from build123d import *

# Parameters (mm, degrees)
SKETCH2_R           = 1.4
SKETCH2_R_2         = 1.65
BOSS_EXTRUDE1_DEPTH = 4.7
SKETCH3_R           = 4.5
SKETCH3_R_2         = 1.65
BOSS_EXTRUDE2_DEPTH = 2
FILLET1_R           = 5
CHAMFER1_SIZE       = 3
CUT_EXTRUDE1_DEPTH  = 3
BOSS_EXTRUDE3_START = -4.7
SKETCH5_R           = 1.4
BOSS_EXTRUDE3_DEPTH = 4.7
BOSS_EXTRUDE4_START = 2.7
SKETCH6_W           = 17.015251106
SKETCH6_H           = 6.441411174
SKETCH6_R           = 1.4
BOSS_EXTRUDE4_DEPTH = 2.7


with BuildPart() as part:
    # Sketch2 → Boss-Extrude1 (new body)
    with BuildSketch(Plane.XY):
        with BuildLine():
            Line((5.681498191, -33.388801204), (5.681498191, -42.638801204))
            Line((5.681498191, -42.638801204), (-15.818501809, -42.638801204))
            Line((-15.818501809, -42.638801204), (-15.818501809, -40.088801204))
            ThreePointArc((-15.818501809, -40.088801204), (-17.282967903, -36.553267298), (-20.818501809, -35.088801204))
            Line((-20.818501809, -35.088801204), (-32.818501809, -35.088801204))
            Line((-32.818501809, -35.088801204), (-32.818501809, -4.488801204))
            Line((-32.818501809, -4.488801204), (-12.818501809, -4.488801204))
            Line((-12.818501809, -4.488801204), (-3.637114605, -4.488801204))
            Line((-3.637114605, -4.488801204), (-3.637114605, -4.888801204))
            Line((-3.637114605, -4.888801204), (-3.637114605, -9.488801204))
            Line((-3.637114605, -9.488801204), (-3.637114605, -33.388801204))
            Line((-3.637114605, -33.388801204), (5.681498191, -33.388801204))
        make_face()
        with Locations((-8.237114605, -14.488801204)):
            Circle(SKETCH2_R, mode=Mode.SUBTRACT)
        with Locations((0.681498191, -37.638801204)):
            Circle(SKETCH2_R_2, mode=Mode.SUBTRACT)
        with BuildLine():
            ThreePointArc((-27.418501809, -27.538801204), (-26.510532831, -29.730832226), (-24.318501809, -30.638801204))
            ThreePointArc((-24.318501809, -30.638801204), (-22.126470787, -25.346770182), (-27.418501809, -27.538801204))
        make_face(mode=Mode.SUBTRACT)
        with BuildLine():
            ThreePointArc((-13.418501809, -27.538801204), (-12.510532831, -29.730832226), (-10.318501809, -30.638801204))
            ThreePointArc((-10.318501809, -30.638801204), (-8.126470787, -25.346770182), (-13.418501809, -27.538801204))
        make_face(mode=Mode.SUBTRACT)
    extrude(amount=BOSS_EXTRUDE1_DEPTH)

    # Sketch3 → Boss-Extrude2 (add)
    # profile 1 of 2: a face of its own
    with BuildSketch(Plane.XY.offset(4.7)):
        with Locations((-24.318501809, -27.538801204)):
            Circle(SKETCH3_R)
        with Locations((-24.318501809, -27.538801204)):
            Circle(SKETCH3_R_2, mode=Mode.SUBTRACT)
    # profile 2 of 2: a face of its own
    with BuildSketch(Plane.XY.offset(4.7)):
        with Locations((-10.318501809, -27.538801204)):
            Circle(SKETCH3_R)
        with Locations((-10.318501809, -27.538801204)):
            Circle(SKETCH3_R_2, mode=Mode.SUBTRACT)
    extrude(amount=BOSS_EXTRUDE2_DEPTH)

    # Fillet1
    fillet1_edges = [part.edges().sort_by_distance(p)[0] for p in [
        (-15.818501809, -42.638801204, 2.35),
        (-32.818501809, -35.088801204, 2.35),
        (-32.818501809, -4.488801204, 2.35),
    ]]
    fillet(fillet1_edges, radius=FILLET1_R)

    # Chamfer1
    chamfer1_edges = [part.edges().sort_by_distance(p)[0] for p in [
        (5.681498191, -33.388801204, 2.35),
        (5.681498191, -42.638801204, 2.35),
    ]]
    chamfer(chamfer1_edges, length=CHAMFER1_SIZE)

    # Sketch4 → Cut-Extrude1 (cut)
    with BuildSketch(Plane.XY.offset(4.7)):
        Polygon((-3.637114605, -42.638801204), (2.681498191, -42.638801204), (5.681498191, -39.638801204), (5.681498191, -36.388801204), (2.681498191, -33.388801204), (-3.637114605, -33.388801204), align=None)
        Polygon((-3.637114605, -9.488801204), (-10.237114605, -9.488801204), (-13.237114605, -12.488801204), (-13.237114605, -16.488801204), (-10.237114605, -19.488801204), (-3.637114605, -19.488801204), align=None)
    extrude(amount=-CUT_EXTRUDE1_DEPTH, mode=Mode.SUBTRACT)

    # Sketch5 → Boss-Extrude3 (add)
    with BuildSketch(Plane(origin=(0, 0, 0), x_dir=(-1, 0, 0), z_dir=(0, 0, -1)).offset(BOSS_EXTRUDE3_START)):
        with BuildLine():
            Line((12.803250703, -4.488801204), (12.803250703, 3.75260997))
            Line((12.803250703, 3.75260997), (30.118597337, 3.75260997))
            Line((30.118597337, 3.75260997), (32.818501809, -2.119551062))
            Line((32.818501809, -2.119551062), (32.818501809, -9.488801204))
            ThreePointArc((32.818501809, -9.488801204), (31.354035715, -5.953267298), (27.818501809, -4.488801204))
            Line((27.818501809, -4.488801204), (12.803250703, -4.488801204))
        make_face()
        with Locations((26.568501809, 1.011198796)):
            Circle(SKETCH5_R, mode=Mode.SUBTRACT)
        with Locations((16.068501809, 1.011198796)):
            Circle(SKETCH5_R, mode=Mode.SUBTRACT)
    extrude(amount=BOSS_EXTRUDE3_DEPTH)

    # Sketch6 → Boss-Extrude4 (add)
    with BuildSketch(Plane.XY.offset(4.7).offset(BOSS_EXTRUDE4_START)):
        with Locations((-21.310876256, 0.531904383)):
            Rectangle(SKETCH6_W, SKETCH6_H)
        with Locations(Location((-26.568501809, 1.011198796, 0), (0, 0, 180))):
            Circle(SKETCH6_R, mode=Mode.SUBTRACT)
        with Locations(Location((-16.068501809, 1.011198796, 0), (0, 0, 180))):
            Circle(SKETCH6_R, mode=Mode.SUBTRACT)
    extrude(amount=-BOSS_EXTRUDE4_DEPTH)


solid = part.part
Check sheet for the modelled part. Datum: model origin and axes. Units: mm. A direction names the side the tool comes from. Give positions to 0.01 mm unless a question says otherwise; leave off trailing zeros. Loops run counter-clockwise (first coordinate to the right, second up) from the corner with the lowest first, then second, coordinate; pieces in that order, holes last. Notation, with made-up numbers: M 38,22.25 L 81,22.25 A27 cw 81,61.25 Z; hole C 17,34.5 d6. An arc over 180 degrees is marked long. Return JSON: item names as keys, results as strings. Group by question number.
1. Cross-section at C-C on y = -6. Record the boundary of the cut face in (x, z).
2. Thickness scan on L1, parallel to X at y = 1.5, z = 4.25; L2, parallel to X at y = -29, z = 4.75; L3, parallel to Y at x = -13, z = 3. Record the ranges inside material, lowest first.
3. Go/stop test with flat-tipped pins: pin 1 (10 mm diameter, centred on x = -5.5, y = -4, fed in from -Z); pin 2 (2.5 mm diameter, centred on x = -24, y = -29.5, fed in from +Z); pin 3 (3 mm diameter, centred on y = -21, z = 5, fed in from +X); pin 4 (4 mm diameter, centred on x = -24, z = 1.5, fed in from -Y). Record where each tip stops, or that it passes through.
4. Tool access check on faces 4 (the flat face through (-11.72, -10.97, 3.22)), 5 (the flat face through (-12.803, 0, 4)), 6 (the flat face through (-24, -35.089, 2)), 7 (the flat face through (2, -39, 1.7)), 8 (the flat face through (-23, -29, 4.7)). Record the directions out of +Z, -Z, +X, -X, +Y, -Y that give a thin tool (end or side, any length) a straight path to the whole face; none if there is none.
5. Cross-section at A-A on y = -37. Record the boundary of the cut face in (x, z), plus the area to 3 significant figures.
6. Cross-section at D-D on z = 3.25. State how many separate pieces and enclosed holes the cut face has, plus the area to 3 significant figures.
7. Cross-section at B-B on x = -3. Record the boundary of the cut face in (y, z), plus the area to 3 significant figures.
8. Mould release check, pull along Y, two halves, no side actions. Record for faces 1 (the flat face through (-7, -9.489, 3)), 2 (the flat face through (-22, -27, 6.7)), 3 (the flat face through (-31.45, 0.86, 2.38)): released by +Y, released by -Y, zero draft, split by the parting line, or undercut.
Return value:
{
 "1": {"outline": "M -32.82,0 L -3.64,0 L -3.64,4.7 L -32.82,4.7 Z"},
 "2": {"L1": "-31.15 to -27.88, -25.26 to -17.38, -14.76 to -12.8", "L2": "-28.57 to -25.08, -23.55 to -20.06, -14.57 to -11.08, -9.55 to -6.06", "L3": "-42.27 to -29.09, -25.98 to -16.73, -12.25 to 3.75"},
 "3": {"pin 1": "z = 0", "pin 2": "z = 6.7", "pin 3": "x = -3.64", "pin 4": "y = -35.09"},
 "4": {"face 4": "+Z, +X", "face 5": "+Z, -Z, +X, +Y", "face 6": "+Z, -Z, -X, -Y", "face 7": "+Z, +X, +Y, -Y", "face 8": "-Z"},
 "5": {"outline": "M -16.89,0 L -0.84,0 L -0.84,1.7 L -3.64,1.7 L -3.64,4.7 L -16.89,4.7 Z; M 2.2,0 L 5.68,0 L 5.68,1.7 L 2.2,1.7 Z", "area": "72.9 mm^2"},
 "6": {"separate pieces": "1", "enclosed holes": "4", "area": "978 mm^2"},
 "7": {"outline": "M -42.64,0 L -33.39,0 L -33.39,1.7 L -42.64,1.7 Z", "area": "15.7 mm^2"},
 "8": {"face 1": "undercut", "face 2": "zero draft", "face 3": "released by +Y"}
}
